Verification items for the finished model (mm, model axes). A direction names the side the tool comes from. Round coordinates to 2 decimals unless told otherwise and drop trailing zeros. Loops run counter-clockwise (first coordinate to the right, second up) from the corner with the lowest first, then second, coordinate; pieces in that order, holes last.
from build123d import *

# Parameters (mm, degrees)
F0_W     = 114.3
F0_H     = 31.75
F1_DEPTH = 63.5
F2_W     = 25.4
F2_H     = 50.8
F2_H_2   = 33.3248
F2_W_2   = 34.925
F2_H_3   = 17.4752
F3_DEPTH = 31.751
F4_R     = 6.35
F5_DEPTH = 88.901
F6_R     = 5.5372
F7_DEPTH = 12.701
F9_DEPTH = 88.901
F10_SIZE = 9.525


with BuildPart() as f1:
    # F0 (on Top) → F1 (new body)
    with BuildSketch(Plane.XY):
        with Locations((44.4766530171, -5.4535213858)):
            Rectangle(F0_W, F0_H)
    extrude(amount=F1_DEPTH)

    # F2 (on face) → F3 (cut, through all)
    with BuildSketch(Plane.XZ.offset(21.3285213858)):
        with Locations((0.0266530171, 38.1)):
            Rectangle(F2_W, F2_H)
        with Locations((44.4766530171, 46.8376)):
            Rectangle(F2_W, F2_H_2)
        with Locations((88.9266530171, 38.1)):
            Rectangle(F2_W, F2_H)
        with Locations((44.4639530171, 8.7376)):
            Rectangle(F2_W_2, F2_H_3)
    extrude(amount=-F3_DEPTH, mode=Mode.SUBTRACT)

    # F4 (on face) → F5 (cut, through all)
    with BuildSketch(Plane.YZ.offset(76.2266530171)):
        with Locations((-5.4535213858, 46.0502)):
            Circle(F4_R)
    extrude(amount=-F5_DEPTH, mode=Mode.SUBTRACT)

    # F6 (on face) → F7 (cut, through all)
    with BuildSketch(Plane.XY.offset(12.7)):
        with Locations((0.0266530171, -2.2785213858)):
            Circle(F6_R)
        with Locations((88.9266530171, -2.2785213858)):
            Circle(F6_R)
    extrude(amount=-F7_DEPTH, mode=Mode.SUBTRACT)

    # F8 (on face) → F9 (cut, through all)
    with BuildSketch(Plane.YZ.offset(76.2266530171)):
        with BuildLine():
            Line((-21.3285213858, 63.5), (-21.3285213858, 59.6835197333))
            ThreePointArc((-21.3285213858, 59.6835197333), (-13.6171777345, 62.5324784108), (-5.4535211745, 63.5))
            Line((-5.4535211745, 63.5), (-21.3285213858, 63.5))
        make_face()
        with BuildLine():
            ThreePointArc((-5.4535211745, 63.5), (2.7101351683, 62.5324783614), (10.4214786142, 59.6835197333))
            Line((10.4214786142, 59.6835197333), (10.4214786142, 63.5))
            Line((10.4214786142, 63.5), (-5.4535211745, 63.5))
        make_face()
    extrude(amount=-F9_DEPTH, mode=Mode.SUBTRACT)

    # F10
    f10_edges = [f1.edges().sort_by_distance(p)[0] for p in [
        (101.626653, -21.328521, 6.35),
        (-12.673347, -21.328521, 6.35),
    ]]
    chamfer(f10_edges, length=F10_SIZE)


solid = f1.part
1. Section check D-D (x = 3). Enter the section's corners in (y, z), then the cut area to 3 significant figures.
2. Section check B-B (z = 9). Enter the section's corners in (x, y).
3. Gauge pin test, flat ends, axial feed: P1, Ø3, axis at x = 20, y = -17.5, coming from the +Z side; P2, Ø12.5, axis at x = 0.03, y = -2.28, coming from the +Z side; P3, Ø16, axis at x = 43.5, y = -2.5, coming from the -Z side. Record the tip position at first contact, or that the pin passes through.
4. Release check for a two-part mould opening along Z. For faces 1 (the face through (89, -9, 12.7)), 2 (the face through (22.39, -6.83, 39.85)), 3 (the face through (81, -5, 0)), 4 (the face through (44, 10.421, 23)) record: released by +Z, released by -Z, zero draft, split by the parting line, or undercut.
5. Section check C-C (x = 21.5). Enter the section's corners in (y, z) (3 decimals).
6. Scan lines: L1, parallel to X at y = 8, z = 33.5; L2, parallel to Y at x = 89, z = 6; L3, parallel to X at y = -3, z = 16. Record each from-to range of solid material in increasing order.
7. Tool access check on faces 5 (the face through (96.93, -16.5, 6.26)), 6 (the face through (12.727, -6, 38)), 7 (the face through (-7.844, -16.633, 6.261)), 8 (the face through (44, -6, 30.175)), 9 (the face through (61.926, -6, 9)). Record the directions out of +Z, -Z, +X, -X, +Y, -Y that give a thin tool (end or side, any length) a straight path to the whole face; none if there is none.
8. Section check A-A (z = 58). Enter the section's corners in (x, y).
Taken from the geometry:
1. outline: (-21.33, 0) - (-6.95, 0) - (-6.95, 12.7) - (-21.33, 12.7) - close; (2.39, 0) - (10.42, 0) - (10.42, 12.7) - (2.39, 12.7) - close
1. area: 285 mm2
2. outline: (-12.67, -11.8) - (-3.15, -21.33) - (27, -21.33) - (27, 10.42) - (-12.67, 10.42) - close; (61.93, -21.33) - (92.1, -21.33) - (101.63, -11.8) - (101.63, 10.42) - (61.93, 10.42) - close; hole circle Ø11.07 at (0.03, -2.28); hole circle Ø11.07 at (88.93, -2.28)
3. P1: stops at z = 61.87
3. P2: stops at z = 12.7
3. P3: stops at z = 17.48
4. face 1: released by +Z
4. face 2: undercut
4. face 3: released by -Z
4. face 4: zero draft
5. outline: (-21.329, 0) - (10.421, 0) - (10.421, 59.684) arc R34.925 ccw to (-21.329, 59.684) - close; hole circle Ø12.7 at (-5.454, 46.05)
6. L1: x = 12.73 to 31.78, 57.18 to 76.23
6. L2: y = -21.33 to -7.82, 3.26 to 10.42
6. L3: x = 12.73 to 27, 61.93 to 76.23
7. face 5: +Z, -Z, +X, -Y
7. face 6: +Z, -X, +Y, -Y
7. face 7: +Z, -Z, -X, -Y
7. face 8: +Z, +Y, -Y
7. face 9: -Z, +Y, -Y
8. outline: (12.73, -21.33) - (31.78, -21.33) - (31.78, 10.42) - (12.73, 10.42) - close; (57.18, -21.33) - (76.23, -21.33) - (76.23, 10.42) - (57.18, 10.42) - close
